Could you check a few things on this model? Use its own coordinates, in mm. Face numbers are marked on the shaded views. Round coordinates to 2 decimals unless told otherwise and drop trailing zeros. Write each loop counter-clockwise with the first axis right and the second up, starting at its lowest first coordinate (ties: lowest second). Pieces come first, ordered by that corner, then holes. Notation, with made-up numbers: (22, 67) - (70, 67) arc R15 cw to (70, 82) - close; hole circle Ø9 at (61.25, -18). An arc over 180 degrees is marked (long way). Put each result on its own line as item: value.
from build123d import *

# Parameters (mm, degrees)
SKETCH1_W               = 40.2
SKETCH1_H               = 40.2
BOSS_EXTRUDE1_DEPTH     = 3
SHELL1_T                = -0.2
SKETCH2_R               = 0.75
HOLES_DEPTH             = 29.583561709
FINGER_START            = 19.9
SKETCH3_W               = 0.5
SKETCH3_H               = 3
FINGER_SLOT_DEPTH       = 0.2
LPATTERN3_COUNT         = 6
LPATTERN3_PITCH         = 6
CIRPATTERN1_START       = -20.1
CIRPATTERN1_OUTLINE_W   = 0.5
CIRPATTERN1_OUTLINE_H   = 3
CIRPATTERN1_DEPTH       = 0.2
CIRPATTERN1_START_2     = 19.9
CIRPATTERN1_2_OUTLINE_W = 0.5
CIRPATTERN1_2_OUTLINE_H = 3
CIRPATTERN1_2_DEPTH     = 0.2
CIRPATTERN1_START_3     = -15.5
CIRPATTERN1_3_OUTLINE_W = 0.2
CIRPATTERN1_3_OUTLINE_H = 3
CIRPATTERN1_3_DEPTH     = 0.5
CIRPATTERN1_START_4     = -9.5
CIRPATTERN1_4_OUTLINE_W = 0.2
CIRPATTERN1_4_OUTLINE_H = 3
CIRPATTERN1_4_DEPTH     = 0.5
CIRPATTERN1_START_5     = -3.5
CIRPATTERN1_5_OUTLINE_W = 0.2
CIRPATTERN1_5_OUTLINE_H = 3
CIRPATTERN1_5_DEPTH     = 0.5
CIRPATTERN1_START_6     = 2.5
CIRPATTERN1_6_OUTLINE_W = 0.2
CIRPATTERN1_6_OUTLINE_H = 3
CIRPATTERN1_6_DEPTH     = 0.5
CIRPATTERN1_START_7     = 8.5
CIRPATTERN1_7_OUTLINE_W = 0.2
CIRPATTERN1_7_OUTLINE_H = 3
CIRPATTERN1_7_DEPTH     = 0.5
CIRPATTERN1_START_8     = 14.5
CIRPATTERN1_8_OUTLINE_W = 0.2
CIRPATTERN1_8_OUTLINE_H = 3
CIRPATTERN1_8_DEPTH     = 0.5


# Read off the part's stored shape, not the designer's step: CirPattern1
with BuildPart() as part:
    # Sketch1 → Boss-Extrude1 (new body)
    with BuildSketch(Plane(origin=(0, 0, 0), x_dir=(1, 0, 0), z_dir=(0, 1, 0))):
        Rectangle(SKETCH1_W, SKETCH1_H)
    extrude(amount=BOSS_EXTRUDE1_DEPTH)

    # Shell1
    shell1_openings = [part.faces().sort_by_distance(p)[0] for p in [
        (0, 0, 0),
    ]]
    offset(amount=SHELL1_T, openings=shell1_openings, kind=Kind.INTERSECTION)

    # Sketch2 → Holes (cut, through all)
    with BuildSketch(Plane(origin=(0, 0, 0), x_dir=(1, 0, 0), z_dir=(0, 1, 0))):
        with Locations(Location((-17.15, -17.15, 0), (0, 0, 90))):
            Circle(SKETCH2_R)
        with Locations(Location((17.15, 17.15, 0), (0, 0, 90))):
            Circle(SKETCH2_R)
    extrude(amount=HOLES_DEPTH, mode=Mode.SUBTRACT)

    # Sketch3 → Finger Slot (cut)
    with BuildSketch(Plane(origin=(0, 0, 0), x_dir=(0, 0, -1), z_dir=(1, 0, 0)).offset(FINGER_START)):
        with Locations((14.75, 1.5)):
            Rectangle(SKETCH3_W, SKETCH3_H)
    finger_slot = extrude(amount=FINGER_SLOT_DEPTH, mode=Mode.SUBTRACT)

    # LPattern3: Finger Slot ×6
    with Locations(*[(0, 0, i * LPATTERN3_PITCH) for i in range(1, LPATTERN3_COUNT)]):
        add(finger_slot, mode=Mode.SUBTRACT)

    # CirPattern1 outline → CirPattern1 (cut)
    with BuildSketch(Plane.XY.offset(CIRPATTERN1_START)):
        with Locations((9.25, 1.5)):
            Rectangle(CIRPATTERN1_OUTLINE_W, CIRPATTERN1_OUTLINE_H)
        with Locations((15.25, 1.5)):
            Rectangle(CIRPATTERN1_OUTLINE_W, CIRPATTERN1_OUTLINE_H)
        with Locations((3.25, 1.5)):
            Rectangle(CIRPATTERN1_OUTLINE_W, CIRPATTERN1_OUTLINE_H)
        with Locations((-2.75, 1.5)):
            Rectangle(CIRPATTERN1_OUTLINE_W, CIRPATTERN1_OUTLINE_H)
        with Locations((-8.75, 1.5)):
            Rectangle(CIRPATTERN1_OUTLINE_W, CIRPATTERN1_OUTLINE_H)
        with Locations((-14.75, 1.5)):
            Rectangle(CIRPATTERN1_OUTLINE_W, CIRPATTERN1_OUTLINE_H)
    extrude(amount=CIRPATTERN1_DEPTH, mode=Mode.SUBTRACT)

    # CirPattern1 2 outline → CirPattern1 2 (cut)
    with BuildSketch(Plane.XY.offset(CIRPATTERN1_START_2)):
        with Locations((14.75, 1.5)):
            Rectangle(CIRPATTERN1_2_OUTLINE_W, CIRPATTERN1_2_OUTLINE_H)
        with Locations((8.75, 1.5)):
            Rectangle(CIRPATTERN1_2_OUTLINE_W, CIRPATTERN1_2_OUTLINE_H)
        with Locations((2.75, 1.5)):
            Rectangle(CIRPATTERN1_2_OUTLINE_W, CIRPATTERN1_2_OUTLINE_H)
        with Locations((-3.25, 1.5)):
            Rectangle(CIRPATTERN1_2_OUTLINE_W, CIRPATTERN1_2_OUTLINE_H)
        with Locations((-9.25, 1.5)):
            Rectangle(CIRPATTERN1_2_OUTLINE_W, CIRPATTERN1_2_OUTLINE_H)
        with Locations((-15.25, 1.5)):
            Rectangle(CIRPATTERN1_2_OUTLINE_W, CIRPATTERN1_2_OUTLINE_H)
    extrude(amount=CIRPATTERN1_2_DEPTH, mode=Mode.SUBTRACT)

    # CirPattern1 3 outline → CirPattern1 3 (cut)
    with BuildSketch(Plane.XY.offset(CIRPATTERN1_START_3)):
        with Locations((-20, 1.5)):
            Rectangle(CIRPATTERN1_3_OUTLINE_W, CIRPATTERN1_3_OUTLINE_H)
    extrude(amount=CIRPATTERN1_3_DEPTH, mode=Mode.SUBTRACT)

    # CirPattern1 4 outline → CirPattern1 4 (cut)
    with BuildSketch(Plane.XY.offset(CIRPATTERN1_START_4)):
        with Locations((-20, 1.5)):
            Rectangle(CIRPATTERN1_4_OUTLINE_W, CIRPATTERN1_4_OUTLINE_H)
    extrude(amount=CIRPATTERN1_4_DEPTH, mode=Mode.SUBTRACT)

    # CirPattern1 5 outline → CirPattern1 5 (cut)
    with BuildSketch(Plane.XY.offset(CIRPATTERN1_START_5)):
        with Locations((-20, 1.5)):
            Rectangle(CIRPATTERN1_5_OUTLINE_W, CIRPATTERN1_5_OUTLINE_H)
    extrude(amount=CIRPATTERN1_5_DEPTH, mode=Mode.SUBTRACT)

    # CirPattern1 6 outline → CirPattern1 6 (cut)
    with BuildSketch(Plane.XY.offset(CIRPATTERN1_START_6)):
        with Locations((-20, 1.5)):
            Rectangle(CIRPATTERN1_6_OUTLINE_W, CIRPATTERN1_6_OUTLINE_H)
    extrude(amount=CIRPATTERN1_6_DEPTH, mode=Mode.SUBTRACT)

    # CirPattern1 7 outline → CirPattern1 7 (cut)
    with BuildSketch(Plane.XY.offset(CIRPATTERN1_START_7)):
        with Locations((-20, 1.5)):
            Rectangle(CIRPATTERN1_7_OUTLINE_W, CIRPATTERN1_7_OUTLINE_H)
    extrude(amount=CIRPATTERN1_7_DEPTH, mode=Mode.SUBTRACT)

    # CirPattern1 8 outline → CirPattern1 8 (cut)
    with BuildSketch(Plane.XY.offset(CIRPATTERN1_START_8)):
        with Locations((-20, 1.5)):
            Rectangle(CIRPATTERN1_8_OUTLINE_W, CIRPATTERN1_8_OUTLINE_H)
    extrude(amount=CIRPATTERN1_8_DEPTH, mode=Mode.SUBTRACT)


solid = part.part
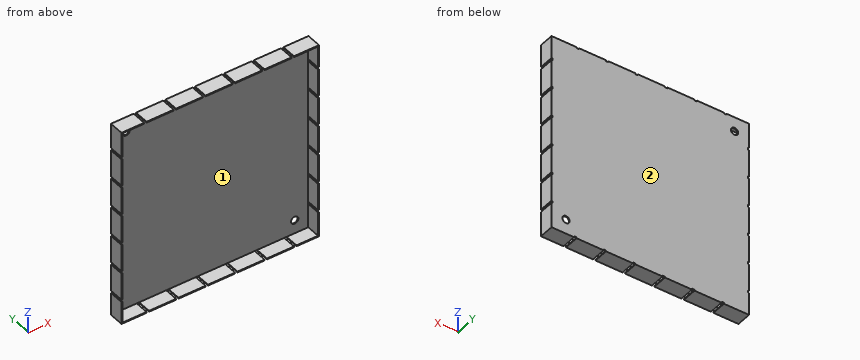
(1) Please list where these lines run through material, in increasing order: probe 1 along Z at (x, y) = (5, 2.1); probe 2 along X at (y, z) = (2.95, -17.15). Write a range as from..to.
Values found:
probe 1: z = -20.1..-19.9, 19.9..20.1
probe 2: x = -20.1..16.4, 17.9..20.1
(2) Imagine slicing it at D-D, the plane z = 1.5. List the corners of the cut face in (x, y) for me, then the cut area to 3 significant figures.
Values found:
outline: (-20.1, 0) - (-19.9, 0) - (-19.9, 2.8) - (19.9, 2.8) - (19.9, 0) - (20.1, 0) - (20.1, 3) - (-20.1, 3) - close
area: 9.16 mm^2
(3) Imagine slicing it at B-B, the plane x = 17.15. List the corners of the cut face in (y, z) for me, then the cut area to 3 significant figures.
Values found:
outline: (0, -20.1) - (3, -20.1) - (3, -17.9) - (2.8, -17.9) - (2.8, -19.9) - (0, -19.9) - close; (0, 19.9) - (2.8, 19.9) - (2.8, -16.4) - (3, -16.4) - (3, 20.1) - (0, 20.1) - close
area: 8.86 mm^2
(4) If we mould it in two halves opening along Z, with no side actions, what happens to the marked faces 1 and 2? For each: pulls with the +Z half, pulls with the -Z half, needs draft (parallel to the pull), parting line crosses it, or undercut.
Values found:
face 1: undercut
face 2: needs draft
(5) Imagine slicing it at A-A, the plane z = 17.15. List the corners of the cut face in (x, y) for me.
Values found:
outline: (-20.1, 0) - (-19.9, 0) - (-19.9, 2.8) - (-17.9, 2.8) - (-17.9, 3) - (-20.1, 3) - close; (-16.4, 2.8) - (19.9, 2.8) - (19.9, 0) - (20.1, 0) - (20.1, 3) - (-16.4, 3) - close
(6) Imagine slicing it at C-C, the plane x = 2. List the corners of the cut face in (y, z) for me, then the cut area to 3 significant figures.
Values found:
outline: (0, -20.1) - (3, -20.1) - (3, 20.1) - (0, 20.1) - (0, 19.9) - (2.8, 19.9) - (2.8, -19.9) - (0, -19.9) - close
area: 9.16 mm^2
